```python
from build123d import *

# Parameters (mm, degrees)
SKETCH1_W           = 100
SKETCH1_H           = 60
BOSS_EXTRUDE1_DEPTH = 10
BOSS_EXTRUDE2_DEPTH = 100
SKETCH3_W           = 100
SKETCH3_H           = 63.245553203
SKETCH3_W_2         = 90
SKETCH3_H_2         = 53.245553203
BOSS_EXTRUDE3_DEPTH = 6
FILLET1_R           = 10
FILLET3_R           = 10


with BuildPart() as part:
    # Sketch1 → Boss-Extrude1 (new body)
    with BuildSketch(Plane(origin=(0, 0, 0), x_dir=(0, 0, -1), z_dir=(1, 0, 0))):
        Rectangle(SKETCH1_W, SKETCH1_H)
    extrude(amount=BOSS_EXTRUDE1_DEPTH)

    # Sketch2 → Boss-Extrude2 (add)
    with BuildSketch(Plane.XY.offset(50)):
        Polygon((10, 30), (30, -30), (10, -30), align=None)
    extrude(amount=-BOSS_EXTRUDE2_DEPTH)

    # Sketch3 → Boss-Extrude3 (add)
    with BuildSketch(Plane(origin=(18, 6, 0), x_dir=(0, 0, -1), z_dir=(0.9486832980505139, 0.316227766016838, 0))):
        with Locations((0, -6.324555321)):
            Rectangle(SKETCH3_W, SKETCH3_H)
        with Locations((0, -6.324555321)):
            Rectangle(SKETCH3_W_2, SKETCH3_H_2, mode=Mode.SUBTRACT)
    extrude(amount=BOSS_EXTRUDE3_DEPTH)

    # Fillet1
    # the kernel refuses this fillet: 10 mm, written as the material it takes off along each edge
    with BuildSketch(Plane(origin=(15.692099788, 31.897366596, 72.912878475), x_dir=(0.31622776601683805, -0.9486832980505137, 0), z_dir=(0, 0, -1))) as fillet1_piece_1:
        with BuildLine():
            CenterArc((9.16515139, 10), FILLET1_R, 203.578178478, 66.421821522)
            Line((0, 6), (0, 0))
            Line((0, 0), (9.16515139, 0))
        make_face()
    extrude(amount=145.82575695, mode=Mode.SUBTRACT)

    # Fillet3
    # the kernel refuses this fillet: 10 mm, written as the material it takes off along each edge
    with BuildSketch(Plane(origin=(35.692099788, -28.102633404, -72.912878475), x_dir=(-0.9486832980505142, -0.3162277660168365, 0), z_dir=(0, 0, 1))) as fillet3_piece_1:
        with BuildLine():
            CenterArc((10, -9.16515139), FILLET3_R, 113.578178478, 66.421821522)
            Line((0, -9.16515139), (-0.2, -9.16515139))
            Line((-0.2, -9.16515139), (-0.2, 0))
            Line((-0.2, 0), (0, 0.2))
            ThreePointArc((0, 0.2), (3, 0.2), (5.92, 0.183303028))
            Line((5.92, 0.183303028), (6, 0))
        make_face()
    extrude(amount=145.82575695, mode=Mode.SUBTRACT)


solid = part.part
```
Part model, mm, in its own coordinate system. A direction names the side the tool comes from. Coordinates: 2 decimals unless noted, no trailing zeros. Order: outer loops, then holes, each group sorted by start corner. A loop starts at its lowest first (then second) coordinate and runs counter-clockwise, first axis right, second up. Notation, with made-up numbers: (82, 60.25) - (103, 60.25) arc R20 ccw to (103, 96.25) - close; hole circle Ø9 at (54.5, 76.5). An arc over 180 degrees is marked (long way). Return JSON: item names as keys, results as strings. Group by question number.
Item 1: Which spindle directions (+Z, -Z, +X, -X, +Y, -Y) get a long thin tool onto all of the face, cutting with end or side? Do faces 4 (the face through (30.8, -24.463, 0.63)), 5 (the face through (0, 0, 1)). Say none if no direction does.
Item 2: Cut at B-B (y = -5.5). List the corners of the cut face in (x, z), plus the area to 3 significant figures.
Item 3: Drill centre lines: probe 1 along Z at (x, y) = (28, -23); probe 2 along X at (y, z) = (6.5, 11.5); probe 3 along X at (y, z) = (9, 36.5). Where is each one in solid material? Low to high. Write a range as from..to.
Item 4: Cut at A-A (z = -21). List the corners of the cut face in (x, y), plus the area to 3 significant figures.
Item 5: Pull direction Y, two halves, no side cores. Call faces 1 (the face through (13.96, 26.05, 0.63)), 2 (the face through (5, 30, 1)), 3 (the face through (12, -1, 50)): pulls with the +Y half, pulls with the -Y half, needs draft (parallel to the pull), parting line crosses it, or undercut.
Item 6: Pin check, flat tips, straight feed: pin 1 (2 mm diameter, centred on y = 4, z = -16, fed in from -X); pin 2 (3 mm diameter, centred on y = 4, z = 28.5, fed in from +X). Stop position of each tip, or through.
Check values:
{
 "1": {"face 4": "+Y", "face 5": "+Z, -Z, -X, +Y, -Y"},
 "2": {"outline": "(0, -50) - (28.16, -50) - (28.16, -45) - (21.83, -45) - (21.83, 45) - (28.16, 45) - (28.16, 50) - (0, 50) - close", "area": "2,250 mm2"},
 "3": {"probe 1": "z = -50..-45, 45..50", "probe 2": "x = 0..17.83", "probe 3": "x = 0..17"},
 "4": {"outline": "(0, -30) - (30, -30) arc R10 ccw to (33.25, -23.65) - (28.42, -25.26) - (11.58, 25.26) - (16.41, 26.87) arc R10 ccw to (10, 30) - (0, 30) - close", "area": "1,230 mm2"},
 "5": {"face 1": "undercut", "face 2": "pulls with the +Y half", "face 3": "needs draft"},
 "6": {"pin 1": "stops at x = 0", "pin 2": "stops at x = 19.17"}
}
